Geometry check sheet. Reference: the model listing, model coordinates, mm. A direction names the side the tool comes from. Coordinates: 2 decimals unless noted, no trailing zeros. Order: outer loops, then holes, each group sorted by start corner. A loop starts at its lowest first (then second) coordinate and runs counter-clockwise, first axis right, second up.
```python
from build123d import *

# Parameters (mm, degrees)
SKETCH_1_W          = 64.5
SKETCH_1_H          = 45
EXTRUDE_1_DEPTH     = 3
SKETCH_6_W          = 12
SKETCH_6_H          = 10
EXTRUDE_4_DEPTH     = 3
FILLET_1_R          = 2
SKETCH_7_R          = 1.65
CUT_EXTRUDE_3_DEPTH = 6
SKETCH_9_W          = 6
SKETCH_9_H          = 14
CUT_EXTRUDE_4_DEPTH = 10
SKETCH_8_R          = 1.65
CUT_EXTRUDE_5_DEPTH = 10
SKETCH_10_W         = 2.1
SKETCH_10_H         = 10
CUT_EXTRUDE_6_DEPTH = 10
FILLET_2_R          = 1


with BuildPart() as part:
    # 草图1 → 凸台-拉伸1 (new body)
    with BuildSketch(Plane.XY):
        Rectangle(SKETCH_1_W, SKETCH_1_H)
    extrude(amount=EXTRUDE_1_DEPTH)

    # 草图6 → 凸台-拉伸4 (add)
    with BuildSketch(Plane.XY.offset(3)):
        with Locations((32.25, 0)):
            Rectangle(SKETCH_6_W, SKETCH_6_H)
        with Locations((-32.25, 0)):
            Rectangle(SKETCH_6_W, SKETCH_6_H)
    extrude(amount=-EXTRUDE_4_DEPTH)

    # 圆角1
    fillet_1_edges = [part.edges().sort_by_distance(p)[0] for p in [
        (38.25, -5, 1.5),
        (32.25, 5, 1.5),
        (32.25, -5, 1.5),
        (38.25, 5, 1.5),
        (-38.25, 5, 1.5),
        (-32.25, 5, 1.5),
        (-38.25, -5, 1.5),
        (-32.25, -5, 1.5),
        (32.25, -22.5, 1.5),
        (-32.25, -22.5, 1.5),
        (-32.25, 22.5, 1.5),
        (32.25, 22.5, 1.5),
    ]]
    fillet(fillet_1_edges, radius=FILLET_1_R)

    # 草图7 → 切除-拉伸3 (cut)
    with BuildSketch(Plane.XY.offset(3)):
        with Locations((-35.25, 0)):
            Circle(SKETCH_7_R)
        with Locations((35.25, 0)):
            Circle(SKETCH_7_R)
    extrude(amount=-CUT_EXTRUDE_3_DEPTH, mode=Mode.SUBTRACT)

    # 草图9 → 切除-拉伸4 (cut)
    with BuildSketch(Plane.XY.offset(3)):
        with Locations((-35.25, 0)):
            Rectangle(SKETCH_9_W, SKETCH_9_H)
        with Locations((35.25, 0)):
            Rectangle(SKETCH_9_W, SKETCH_9_H)
    extrude(amount=-CUT_EXTRUDE_4_DEPTH, mode=Mode.SUBTRACT)

    # 草图8 → 切除-拉伸5 (cut)
    with BuildSketch(Plane.XY.offset(3)):
        with Locations((-26.25, 0)):
            Circle(SKETCH_8_R)
        with Locations((26.25, 0)):
            Circle(SKETCH_8_R)
    extrude(amount=-CUT_EXTRUDE_5_DEPTH, mode=Mode.SUBTRACT)

    # 草图10 → 切除-拉伸6 (cut)
    with BuildSketch(Plane.XY.offset(3)):
        with Locations((0, -17)):
            Rectangle(SKETCH_10_W, SKETCH_10_H)
    extrude(amount=-CUT_EXTRUDE_6_DEPTH, mode=Mode.SUBTRACT)

    # 圆角2
    fillet_2_edges = [part.edges().sort_by_distance(p)[0] for p in [
        (1.05, -12, 1.5),
        (1.05, -22, 1.5),
        (-1.05, -22, 1.5),
        (-1.05, -12, 1.5),
    ]]
    fillet(fillet_2_edges, radius=FILLET_2_R)


solid = part.part
```
Item 1: Tool access check on faces 1 (the face through (1.05, -17, 2)), 2 (the face through (0, -22.5, 1)). Record the directions out of +Z, -Z, +X, -X, +Y, -Y that give a thin tool (end or side, any length) a straight path to the whole face; none if there is none.
Item 2: Release check for a two-part mould opening along Y. For faces 3 (the face through (-31.68, -21.9, 1.52)), 4 (the face through (-1.05, -17, 2)), 5 (the face through (-32.25, 0, 1)) record: pulls with the +Y half, pulls with the -Y half, needs draft (parallel to the pull), parting line crosses it, or undercut.
Item 3: Depth check by flat-ended pin: P1, Ø4, axis at x = 14.5, y = 0, coming from the -Z side; P2, Ø3, axis at x = 26.25, y = 0, coming from the -Z side. Enter the tip coordinate at first touch or a pass-through.
Item 4: Sectioned sample at A-A (y = 0). Record the cut outline in (x, z).
Item 5: Sectioned sample at B-B (x = 26.25). Record the cut outline in (y, z).
Item 6: Thickness scan on line 1 along Y through (x, z) = (26.25, 0.7); line 2 along X through (y, z) = (-17.5, 1.85); line 3 along X through (y, z) = (0.5, 2.3). Record the ranges inside material, lowest first.
Geometry check:
1. face 1: +Z, -Z
1. face 2: +Z, -Z, +X, -X, -Y
2. face 3: pulls with the -Y half
2. face 4: undercut
2. face 5: needs draft
3. P1: stops at z = 0
3. P2: passes through
4. outline: (-32.25, 0) - (-27.9, 0) - (-27.9, 3) - (-32.25, 3) - close; (-24.6, 0) - (24.6, 0) - (24.6, 3) - (-24.6, 3) - close; (27.9, 0) - (32.25, 0) - (32.25, 3) - (27.9, 3) - close
5. outline: (-22.5, 0) - (-1.65, 0) - (-1.65, 3) - (-22.5, 3) - close; (1.65, 0) - (22.5, 0) - (22.5, 3) - (1.65, 3) - close
6. line 1: y = -22.5 to -1.65, 1.65 to 22.5
6. line 2: x = -32.25 to -1.05, 1.05 to 32.25
6. line 3: x = -32.25 to -27.82, -24.68 to 24.68, 27.82 to 32.25
